Verification items for this drawing (mm, ordinates from the low corner). A direction names the side the tool comes from. Coordinates: 2 decimals unless noted, no trailing zeros. Write each loop counter-clockwise with the first axis right and the second up, starting at its lowest first coordinate (ties: lowest second). Pieces come first, ordered by that corner, then holes. Notation, with made-up numbers: (57, -23.5) -> (108, -23.5) arc R26 ccw to (108, -1.5) -> close; hole circle Ø9 at (67, -18). An arc over 180 degrees is marked (long way). Use CSV: the item, a comma, the result in double quotes.
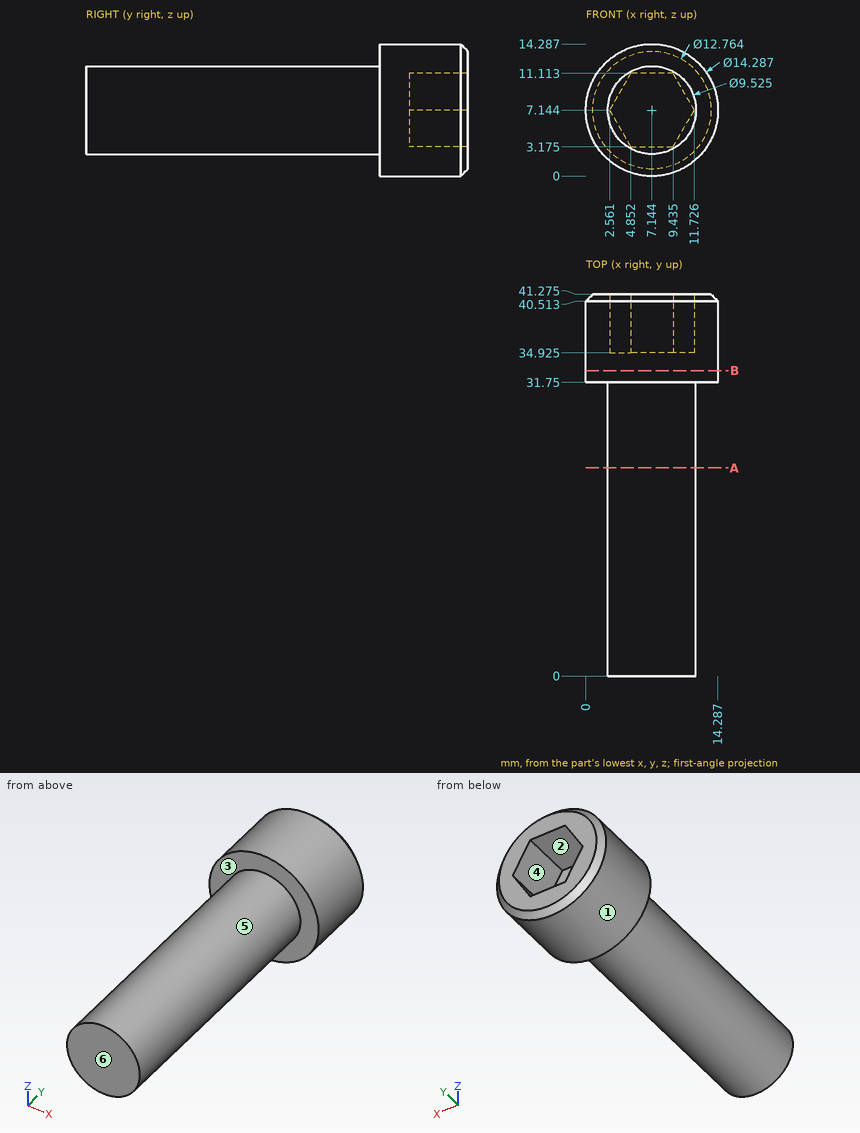
1) Cross-section at A-A (y = 22.5). Record the boundary of the cut face in (x, z) (1 decimal).
Return value:
outline,"circle Ø9.5 at (7.1, 7.1)"
2) Cross-section at B-B (y = 33). Record the boundary of the cut face in (x, z).
Return value:
outline,"circle Ø14.29 at (7.14, 7.14)"
3) Gauge pin test, flat ends, axial feed: pin 1 (4.5 mm diameter, centred on x = 8.5, z = 8.5, fed in from -Y); pin 2 (1 mm diameter, centred on y = 25, z = 12.5, fed in from -X); pin 3 (5 mm diameter, centred on y = 13.5, z = 8, fed in from +X); pin 4 (5 mm diameter, centred on y = 29, z = 3, fed in from -X). Record the tip position at first contact, or that the pin passes through.
Return value:
pin 1,"y = 0"
pin 2,"through"
pin 3,"x = 11.91"
pin 4,"x = 2.67"
4) Set-up check for the marked faces 4, 5 and 6: record each of +Z, -Z, +X, -X, +Y, -Y from which the full face is reachable in a straight line by a thin tool's end or side.
Return value:
face 4,"+Y"
face 5,"-Y"
face 6,"+Z, -Z, +X, -X, -Y"
5) Scan lines: L1, parallel to Y at x = 7, z = 5.5 (1 decimal); L2, parallel to Z at x = 8.5, y = 38 (1 decimal); L3, parallel to X at y = 28, z = 4.5 (1 decimal). Record each from-to range of solid material in increasing order.
Return value:
L1,"0 to 34.9"
L2,"0.1 to 3.2, 11.1 to 14.2"
L3,"3.2 to 11.1"
6) Mould release check, pull along Z, two halves, no side actions. Record for the marked faces 1, 2 and 3: released by +Z, released by -Z, zero draft, split by the parting line, or undercut.
Return value:
face 1,"split by the parting line"
face 2,"undercut"
face 3,"zero draft"
